from build123d import *

# Parameters (mm, degrees)
SKETCH1_W                = 32.26
SKETCH1_H                = 9.678
BOSS_EXTRUDE1_DEPTH      = 8.065
SKETCH2_W                = 28.975
SKETCH2_H                = 4.78
CUT_EXTRUDE1_DEPTH       = 8.0355
BOSS_EXTRUDE2_DEPTH      = 4.78
BOSS_EXTRUDE3_DEPTH      = 4.78
BOSS_EXTRUDE4_DEPTH      = 4.78
SKETCH6_W                = 2.39
SKETCH6_H                = 1.78
SKETCH7_W                = 2.39
SKETCH7_H                = 1.78
SKETCH8_W                = 2.39
SKETCH8_H                = 1.78
SKETCH9_W                = 2.39
SKETCH9_H                = 1.78
SKETCH13_W               = 3.195419505
SKETCH13_H               = 1.6425
SKETCH14_W               = 3.195419505
SKETCH14_H               = 1.6425
SKETCH15_W               = 3.195419505
SKETCH15_H               = 1.6425
M3_CLEARANCE_HOLE1_D     = 3.285
M3_CLEARANCE_HOLE1_DEPTH = 1.78


with BuildPart() as part:
    # Sketch1 → Boss-Extrude1 (new body)
    with BuildSketch(Plane(origin=(0, 4.0325, 0), x_dir=(-1, 0, 0), z_dir=(0, 1, 0))):
        Rectangle(SKETCH1_W, SKETCH1_H)
    extrude(amount=-BOSS_EXTRUDE1_DEPTH)

    # Sketch2 → Cut-Extrude1 (cut)
    with BuildSketch(Plane.XY.offset(4.839)):
        Rectangle(SKETCH2_W, SKETCH2_H)
    extrude(amount=-CUT_EXTRUDE1_DEPTH, mode=Mode.SUBTRACT)

    # Sketch3 → Boss-Extrude2 (add)
    with BuildSketch(Plane.XZ.offset(-2.39)):
        with BuildLine():
            Line((10.171130278, -3.1965), (5.958869722, -3.1965))
            ThreePointArc((5.958869722, -3.1965), (8.065, 2.119), (10.171130278, -3.1965))
        make_face()
    extrude(amount=BOSS_EXTRUDE2_DEPTH)

    # Sketch4 → Boss-Extrude3 (add)
    with BuildSketch(Plane.XZ.offset(-2.39)):
        with BuildLine():
            Line((2.106130278, -3.1965), (-2.106130278, -3.1965))
            ThreePointArc((-2.106130278, -3.1965), (0, 2.119), (2.106130278, -3.1965))
        make_face()
    extrude(amount=BOSS_EXTRUDE3_DEPTH)

    # Sketch5 → Boss-Extrude4 (add)
    with BuildSketch(Plane.XZ.offset(-2.39)):
        with BuildLine():
            Line((-5.958869722, -3.1965), (-10.171130278, -3.1965))
            ThreePointArc((-10.171130278, -3.1965), (-8.065, 2.119), (-5.958869722, -3.1965))
        make_face()
    extrude(amount=BOSS_EXTRUDE4_DEPTH)

    # Sketch6 → Revolve1 (revolve)
    with BuildSketch(Plane.XZ):
        with Locations((13.2925, -5.729)):
            Rectangle(SKETCH6_W, SKETCH6_H)
    revolve(axis=Axis((12.0975, 0, -4.839), (0, 0, -1)))

    # Sketch7 → Revolve2 (revolve)
    with BuildSketch(Plane.XZ):
        with Locations((5.2275, -5.729)):
            Rectangle(SKETCH7_W, SKETCH7_H)
    revolve(axis=Axis((4.0325, 0, -4.839), (0, 0, -1)))

    # Sketch8 → Revolve3 (revolve)
    with BuildSketch(Plane.XZ):
        with Locations((-2.8375, -5.729)):
            Rectangle(SKETCH8_W, SKETCH8_H)
    revolve(axis=Axis((-4.0325, 0, -4.839), (0, 0, -1)))

    # Sketch9 → Revolve4 (revolve)
    with BuildSketch(Plane.XZ):
        with Locations((-10.9025, -5.729)):
            Rectangle(SKETCH9_W, SKETCH9_H)
    revolve(axis=Axis((-12.0975, 0, -4.839), (0, 0, -1)))

    # Sketch10 → Cut-Revolve1 (revolve, cut)
    with BuildSketch(Plane(origin=(0, 0, -0.956), x_dir=(-1, 0, 0), z_dir=(0, 0, -1))):
        Polygon((-11.14, -4.0325), (-8.065, -4.0325), (-8.065, 4.0325), (-11.14, 4.0325), (-11.14, 3.2175), (-10.455, 3.2175), (-10.455, -3.2175), (-11.14, -3.2175), align=None)
    revolve(axis=Axis((8.065, -4.0325, -0.956), (0, 1, 0)), mode=Mode.SUBTRACT)

    # Sketch11 → Cut-Revolve2 (revolve, cut)
    with BuildSketch(Plane(origin=(0, 0, -0.956), x_dir=(-1, 0, 0), z_dir=(0, 0, -1))):
        Polygon((-3.075, -4.0325), (0, -4.0325), (0, 4.0325), (-3.075, 4.0325), (-3.075, 3.2175), (-2.39, 3.2175), (-2.39, -3.2175), (-3.075, -3.2175), align=None)
    revolve(axis=Axis((0, -4.0325, -0.956), (0, 1, 0)), mode=Mode.SUBTRACT)

    # Sketch12 → Cut-Revolve3 (revolve, cut)
    with BuildSketch(Plane(origin=(0, 0, -0.956), x_dir=(-1, 0, 0), z_dir=(0, 0, -1))):
        Polygon((4.99, -4.0325), (8.065, -4.0325), (8.065, 4.0325), (4.99, 4.0325), (4.99, 3.2175), (5.675, 3.2175), (5.675, -3.2175), (4.99, -3.2175), align=None)
    revolve(axis=Axis((-8.065, -4.0325, -0.956), (0, 1, 0)), mode=Mode.SUBTRACT)

    # Sketch13 → Revolve5 (revolve)
    with BuildSketch(Plane(origin=(-8.065, 0, 0), x_dir=(0, 0, -1), z_dir=(1, 0, 0))):
        with Locations((-3.241290248, 0.82125)):
            Rectangle(SKETCH13_W, SKETCH13_H)
    revolve(axis=Axis((-8.065, 0, 4.839), (0, 0, -1)))

    # Sketch14 → Revolve6 (revolve)
    with BuildSketch(Plane(origin=(0, 0, 0), x_dir=(0, 0, -1), z_dir=(1, 0, 0))):
        with Locations((-3.241290248, 0.82125)):
            Rectangle(SKETCH14_W, SKETCH14_H)
    revolve(axis=Axis((0, 0, 4.839), (0, 0, -1)))

    # Sketch15 → Revolve7 (revolve)
    with BuildSketch(Plane(origin=(8.065, 0, 0), x_dir=(0, 0, -1), z_dir=(1, 0, 0))):
        with Locations((-3.241290248, 0.82125)):
            Rectangle(SKETCH15_W, SKETCH15_H)
    revolve(axis=Axis((8.065, 0, 4.839), (0, 0, -1)))

    # M3 Clearance Hole1
    with Locations(Plane(origin=(0, 0, -6.619), x_dir=(-1, 0, 0), z_dir=(0, 0, -1))):
        with Locations((12.0975, 0), (4.0325, 0), (-4.0325, 0), (-12.0975, 0)):
            Hole(M3_CLEARANCE_HOLE1_D / 2, depth=M3_CLEARANCE_HOLE1_DEPTH)


solid = part.part
Could you check a few things on this model? Use its own coordinates, in mm. A direction names the side the tool comes from. Give positions to 0.01 mm unless a question says otherwise; leave off trailing zeros. Order: outer loops, then holes, each group sorted by start corner. A loop starts at its lowest first (then second) coordinate and runs counter-clockwise, first axis right, second up. Notation, with made-up numbers: (37, 48.25) -> (60, 48.25) arc R12 ccw to (60, 69.25) -> close; hole circle Ø5 at (-24, 7.25). An arc over 180 degrees is marked (long way). Return JSON: item names as keys, results as strings.
1. I need wall thicknesses on line 1 (Y direction, x = -14, z = 1.5); line 2 (Z direction, x = -13, y = 0.5); line 3 (Z direction, x = 11.5, y = 3). Which ranges of each line are inside material? Lowest first, please. Write a range as from..to.
Answer list:
{"line 1": "y = -4.03..-2.39, 2.39..4.03", "line 2": "z = -4.84..-3.2", "line 3": "z = -4.84..4.84"}
2. Imagine slicing it at A-A on z = -5.25. List the corners of the cut face in (x, y) for me (1 decimal).
Answer list:
{"outline": "circle Ø4.8 at (-12.1, 0); circle Ø4.8 at (-4, 0); circle Ø4.8 at (4, 0); circle Ø4.8 at (12.1, 0); hole circle Ø3.3 at (-12.1, 0); hole circle Ø3.3 at (-4, 0); hole circle Ø3.3 at (4, 0); hole circle Ø3.3 at (12.1, 0)"}
3. Imagine slicing it at B-B on z = 3.75. List the corners of the cut face in (x, y) for me (1 decimal).
Answer list:
{"outline": "(-16.1, -4) -> (16.1, -4) -> (16.1, 4) -> (-16.1, 4) -> close; circle Ø3.3 at (-8.1, 0); circle Ø3.3 at (0, 0); circle Ø3.3 at (8.1, 0); hole (-14.5, -2.4) -> (14.5, -2.4) -> (14.5, 2.4) -> (-14.5, 2.4) -> close"}
4. Imagine slicing it at C-C on x = 0. List the corners of the cut face in (y, z) for me.
Answer list:
{"outline": "(-4.03, -4.84) -> (4.03, -4.84) -> (4.03, -4.03) -> (3.22, -4.03) -> (3.22, -3.35) -> (-3.22, -3.35) -> (-3.22, -4.03) -> (-4.03, -4.03) -> close; (-4.03, 2.12) -> (-3.22, 2.12) -> (-3.22, 1.43) -> (3.22, 1.43) -> (3.22, 2.12) -> (4.03, 2.12) -> (4.03, 4.84) -> (2.39, 4.84) -> (2.39, 2.12) -> (1.64, 2.12) -> (1.64, 4.84) -> (-1.64, 4.84) -> (-1.64, 2.12) -> (-2.39, 2.12) -> (-2.39, 4.84) -> (-4.03, 4.84) -> close"}
5. On a 3-axis mill with a long thin cutter (end or side, diameter ignored), from which of +Z, -Z, +X, -X, +Y, -Y can I reach the whole of each face in a straight line? I mean faces 1 (the flat face through (-6, 3.218, 1)), 2 (the cylindrical face through (14.377, -0.718, -5.717)), 3 (the flat face through (-12, 0, -3.197)), 4 (the cylindrical face through (-5.132, -3.631, -1.88)). Say none if no direction works.
Answer list:
{"face 1": "+Y", "face 2": "-Z", "face 3": "none", "face 4": "-Y"}
6. For pin 1 Ø5 at (x, z) = (8.065, -0.956) entering from -Y; pin 2 Ø6 at (x, z) = (8.065, -0.956) entering from +Y; pin 3 Ø1.9 at (x, y) = (3.5, -0.5) entering from +Z, each with a flat end and sliding along its axis, tell me the tip position at first contact or that it passes through.
Answer list:
{"pin 1": "stops at y = -3.22", "pin 2": "stops at y = 3.22", "pin 3": "stops at z = 0.76"}
7. Imagine slicing it at D-D on x = 13. List the corners of the cut face in (y, z) for me.
Answer list:
{"outline": "(-4.03, -4.84) -> (-2.21, -4.84) -> (-2.21, -6.62) -> (-1.37, -6.62) -> (-1.37, -4.84) -> (1.37, -4.84) -> (1.37, -6.62) -> (2.21, -6.62) -> (2.21, -4.84) -> (4.03, -4.84) -> (4.03, 4.84) -> (2.39, 4.84) -> (2.39, -3.2) -> (-2.39, -3.2) -> (-2.39, 4.84) -> (-4.03, 4.84) -> close"}
8. Thinking about a two-plate mould opening in Y: for faces 5 (the flat face through (-4, 0, -3.197)), 6 (the flat face through (2, 3.218, 1)), 7 (the flat face through (0, 3, 4.839)), which applies, pulls with the +Y half, pulls with the -Y half, needs draft (parallel to the pull), parting line crosses it, or undercut?
Answer list:
{"face 5": "undercut", "face 6": "pulls with the +Y half", "face 7": "needs draft"}
